```python
from build123d import *

# Parameters (mm, degrees)
F1_DEPTH = 111


with BuildPart() as f1:
    # F0 (on Front) → F1 (new body)
    with BuildSketch(Plane.XZ):
        with BuildLine():
            Line((0, 29), (0, 15))
            Line((0, 15), (19, 15))
            Line((19, 15), (19, 0))
            Line((19, 0), (39, 0))
            ThreePointArc((39, 0), (33.128812, 25.713323), (12, 41.5))
            ThreePointArc((12, 41.5), (4.844107, 36.359658), (0, 29))
        make_face()
    extrude(amount=F1_DEPTH)


solid = f1.part
```
Check sheet for the modelled part. Datum: model origin and axes. Units: mm. A direction names the side the tool comes from. Round coordinates to 2 decimals unless told otherwise and drop trailing zeros. Write each loop counter-clockwise with the first axis right and the second up, starting at its lowest first coordinate (ties: lowest second). Pieces come first, ordered by that corner, then holes. Notation, with made-up numbers: (-2, 73.25) -> (11, 73.25) arc R16 ccw to (11, 104.25) -> close; hole circle Ø4 at (43, -4). An arc over 180 degrees is marked (long way). One line per question, with ' | ' between items. Start each with the question number.
1. Scan lines: line 1 along X through (y, z) = (-61, 5); line 2 along X through (y, z) = (-57, 33.5); line 3 along Z through (x, y) = (36, -94). Record each from-to range of solid material in increasing order. Write a range as from..to.
2. Sectioned sample at B-B, the plane x = 26.5. Record the cut outline in (y, z), then the cut area to 3 significant figures.
3. Sectioned sample at C-C, the plane z = 25. Record the cut outline in (x, y), then the cut area to 3 significant figures.
4. Depth check by flat-ended pin: pin 1 (1.5 mm diameter, centred on y = -87.5, z = 8.5, fed in from +X); pin 2 (15 mm diameter, centred on x = 6.5, y = -60.5, fed in from -Z); pin 3 (5 mm diameter, centred on y = -76.5, z = 35, fed in from -X); pin 4 (1 mm diameter, centred on x = 22.5, y = -65, fed in from -Z). Enter the tip coordinate at first touch or a pass-through.
5. Sectioned sample at A-A, the plane y = -65.5. Record the cut outline in (x, z), then the cut area to 3 significant figures.
6. Set-up check for faces 1 (the face through (19, -55, 8)), 2 (the face through (0, -55, 22)): record each of +Z, -Z, +X, -X, +Y, -Y from which the full face is reachable in a straight line by a thin tool's end or side.
Taken from the geometry:
1) line 1: x = 19..39.31 | line 2: x = 2.49..26.41 | line 3: z = 0..20.43
2) outline: (-111, 0) -> (0, 0) -> (0, 33.42) -> (-111, 33.42) -> close | area: 3,710 mm^2
3) outline: (0, -111) -> (33.58, -111) -> (33.58, 0) -> (0, 0) -> close | area: 3,730 mm^2
4) pin 1: stops at x = 39.2 | pin 2: stops at z = 15 | pin 3: stops at x = 1.83 | pin 4: stops at z = 0
5) outline: (0, 15) -> (19, 15) -> (19, 0) -> (39, 0) arc R38.22 ccw to (12, 41.5) arc R24.22 ccw to (0, 29) -> close | area: 1,030 mm^2
6) face 1: -Z, -X, +Y, -Y | face 2: +Z, -Z, -X, +Y, -Y
